Geometry: final body of the model. Coordinates: model frame, mm. A direction names the side the tool comes from. Coordinates: 2 decimals unless noted, no trailing zeros. Order: outer loops, then holes, each group sorted by start corner. A loop starts at its lowest first (then second) coordinate and runs counter-clockwise, first axis right, second up. Notation, with made-up numbers: M 69.5,-13.75 L 91.5,-13.75 A22 ccw 91.5,11.25 Z; hole C 64,-15.75 d10. An arc over 180 degrees is marked long. Write item = value, one per line.
from build123d import *

# Parameters (mm, degrees)
F1_DEPTH = 10
F2_SIZE  = 2


with BuildPart() as f1:
    # F0 (on Right) → F1 (new body)
    with BuildSketch(Plane.YZ):
        with BuildLine():
            Line((-42.5, 0), (0, 0))
            Line((0, 0), (0, 100))
            Line((0, 100), (11, 100))
            Line((11, 100), (11, 50))
            Line((11, 50), (21, 50))
            Line((21, 50), (21, 110))
            ThreePointArc((21, 110), (5.5, 115.384955), (-10, 110))
            Line((-10, 110), (-10, 60))
            Line((-10, 60), (-20, 10))
            Line((-20, 10), (-85, 10))
            Line((-85, 10), (-85, 20))
            ThreePointArc((-85, 20), (-87.701489, 22.985112), (-90.940594, 20.594059))
            Line((-90.940594, 20.594059), (-94.90099, 0.990099))
            ThreePointArc((-94.90099, 0.990099), (-93.697535, -3.365745), (-89.473684, -4.972222))
            Line((-89.473684, -4.972222), (-42.5, 0))
        make_face()
    extrude(amount=F1_DEPTH)

    # F2
    f2_edges = [f1.edges().sort_by_distance(p)[0] for p in [
        (0, -93.697535, -3.365745),
        (0, -65.986842, -2.486111),
        (0, -21.25, 0),
        (0, 0, 50),
        (0, 5.5, 100),
        (0, 11, 75),
        (0, 16, 50),
        (0, 21, 80),
        (0, 5.5, 115.384955),
        (0, -10, 85),
        (0, -15, 35),
        (0, -52.5, 10),
        (0, -85, 15),
        (0, -87.701489, 22.985112),
        (0, -92.920792, 10.792079),
        (10, -93.697535, -3.365745),
        (10, -65.986842, -2.486111),
        (10, -21.25, 0),
        (10, 0, 50),
        (10, 5.5, 100),
        (10, 11, 75),
        (10, 16, 50),
        (10, 21, 80),
        (10, 5.5, 115.384955),
        (10, -10, 85),
        (10, -15, 35),
        (10, -52.5, 10),
        (10, -85, 15),
        (10, -87.701489, 22.985112),
        (10, -92.920792, 10.792079),
    ]]
    chamfer(f2_edges, length=F2_SIZE)


solid = f1.part
1) Line query: L1, parallel to Y at x = 2.25, z = 65; L2, parallel to Z at x = 6.5, y = -39.5; L3, parallel to Y at x = 4.75, z = 108. Output: solid intervals per line, ascending.
Numbers:
L1 = -10 to 0, 11 to 21
L2 = 0 to 10
L3 = -10 to 21
2) Pin query (flat end, axial travel): pin 1 (3 mm diameter, centred on x = 6, y = 3, fed in from -Z); pin 2 (12 mm diameter, centred on y = -18, z = 28.5, fed in from -X); pin 3 (1.8 mm diameter, centred on x = 4.5, z = 78, fed in from -Y); pin 4 (5 mm diameter, centred on x = 4.5, z = 16.5, fed in from +Y). Return the tip coordinate at first contact, or that it passes through.
Numbers:
pin_1 = 100
pin_2 = 0
pin_3 = -10
pin_4 = 0
3) Mould query, pull axis Y, two halves, no side actions, for faces 1 (the face through (0.986, -91.899, 10.729)), 2 (the face through (5, -88, 23)), 3 (the face through (4.958, 5.734, 115.384)). Classes: pulls with the +Y half, pulls with the -Y half, needs draft (parallel to the pull), parting line crosses it, or undercut.
Numbers:
face_1 = pulls with the -Y half
face_2 = undercut
face_3 = parting line crosses it
4) Section D-D, the plane y = -48. Return loops of the section in (x, z), and give its area (3 significant figures).
Numbers:
outline = M 0,1.43 L 2,-0.58 L 8,-0.58 L 10,1.43 L 10,8 L 8,10 L 2,10 L 0,8 Z
area = 97.8 mm²
5) Section A-A, the plane z = 78.5. Return loops of the section in (x, y), and give its area (3 significant figures).
Numbers:
outline = M 0,-8 L 2,-10 L 8,-10 L 10,-8 L 10,-2 L 8,0 L 2,0 L 0,-2 Z; M 0,13 L 2,11 L 8,11 L 10,13 L 10,19 L 8,21 L 2,21 L 0,19 Z
area = 184 mm²
6) Section C-C, the plane x = 6.25. Return loops of the section in (y, z), and give its area (3 significant figures).
Numbers:
outline = M -94.9,0.99 A5 ccw -89.47,-4.97 L -42.5,0 L 0,0 L 0,100 L 11,100 L 11,50 L 21,50 L 21,110 A25 ccw -10,110 L -10,60 L -20,10 L -85,10 L -85,20 A3 ccw -90.94,20.59 Z
area = 3,240 mm²
7) Set-up query: faces 4 (the face through (5, -22, 0)), 5 (the face through (0.986, -14.075, 34.457)), 6 (the face through (9.014, -14.075, 34.457)), 7 (the face through (5, 11, 75)). Return all of +Z, -Z, +X, -X, +Y, -Y with unobstructed straight access to the full face (end or side cutting, diameter ignored); none if empty.
Numbers:
face_4 = -Z, +X, -X, +Y
face_5 = +Z, -X
face_6 = +Z, +X
face_7 = -Z, +X, -X
8) Section B-B, the plane z = 104.5. Return loops of the section in (x, y), and give its area (3 significant figures).
Numbers:
outline = M 0,-8 L 2,-10 L 8,-10 L 10,-8 L 10,19 L 8,21 L 2,21 L 0,19 Z
area = 302 mm²
